```python
from build123d import *

# Parameters (mm, degrees)
F0_W     = 93.98
F0_H     = 38.1
F0_R     = 6.985
F1_DEPTH = 25.4
F3_D     = 5.5
F4_W     = 12.7
F4_H     = 5.08


with BuildPart() as f1:
    # F0 (on Front) → F1 (new body)
    with BuildSketch(Plane.XZ):
        with Locations((46.99, 19.05)):
            Rectangle(F0_W, F0_H)
        with Locations((15.24, 12.7)):
            Circle(F0_R, mode=Mode.SUBTRACT)
        Polygon((42.0011818976, 10.16), (50.8, 25.4), (59.5988181024, 10.16), align=None, mode=Mode.SUBTRACT)
    extrude(amount=F1_DEPTH)

    # F3 (through all)
    with Locations(Plane.XZ.offset(25.4)):
        with Locations((76.2, 25.4)):
            Hole(F3_D / 2)

    # F4 (on face) → F5 (revolve, cut)
    with BuildSketch(Plane.XY.offset(38.1)):
        with Locations((39.37, -15.24)):
            Rectangle(F4_W, F4_H)
    revolve(axis=Axis((46.99, 0, 38.1), (1, 0, 0)), mode=Mode.SUBTRACT)


solid = f1.part
```
Read the model definition and answer for the solid it produces. Units are mm, in the model's axes. A direction names the side the tool comes from. Coordinates: 2 decimals unless noted, no trailing zeros. Write each loop counter-clockwise with the first axis right and the second up, starting at its lowest first coordinate (ties: lowest second). Pieces come first, ordered by that corner, then holes. Notation, with made-up numbers: (60, 88) - (96, 88) arc R16 cw to (96, 97) - close; hole circle Ø5 at (88.5, 63). An arc over 180 degrees is marked (long way). Answer as a JSON object with one key per item and string values. Group by question number.
1. A cutting plane is placed at B-B (y = -22). Determine the outline of the cut face in (x, z) (3 decimals), plus the area to 3 significant figures.
2. This flat-tipped pin is pushed along its axis until it touches: P1, Ø11, axis at x = 15.24, z = 12.7, coming from the -Y side. Where does it stop, or does it pass through?
3. The mould has two halves that part along Y. Classify faces 4 (the flat face through (46.339, -12.522, 17.673)), 5 (the cylindrical face through (39.46, -9.08, 29.22)), 6 (the flat face through (46, -25.4, 19)), 7 (the cylindrical face through (39.459, -12.71, 25.667)): +Y half, -Y half, draft (parallel to the pull), parting line (faces both ways), or undercut.
4. A cutting plane is placed at A-A (x = 76.2). Determine the outline of the cut face in (y, z), plus the area to 3 significant figures.
5. Consider L1, parallel to Z at x = 15.24, y = -16.5 (3 decimals); L2, parallel to Z at x = 76.2, y = -8.25; L3, parallel to X at y = -9.25, z = 11. Determine where each line is inside the solid, lowest interval first. Write a range as [from, to].
6. A cutting plane is placed at C-C (z = 12.7). Determine the outline of the cut face in (x, y) (3 decimals), plus the area to 3 significant figures.
7. Which of the six approach directions +Z, -Z, +X, -X, +Y, -Y give full straight-line access (tool end or side, diameter ignored) to faces 1 (the flat face through (45.72, -11, 29)), 2 (the flat face through (51, -13, 10.16)), 3 (the flat face through (46, -13, 0))?
8. A cutting plane is placed at D-D (z = 7.5). Determine the outline of the cut face in (x, y).
Worked out:
{
 "1": {"outline": "(0, 0) - (93.98, 0) - (93.98, 38.1) - (0, 38.1) - close; hole circle Ø13.97 at (15.24, 12.7); hole (42.001, 10.16) - (59.599, 10.16) - (50.8, 25.4) - close; hole circle Ø5.5 at (76.2, 25.4)", "area": "3,270 mm²"},
 "2": {"P1": "passes through"},
 "3": {"face 4": "draft", "face 5": "undercut", "face 6": "-Y half", "face 7": "undercut"},
 "4": {"outline": "(-25.4, 0) - (0, 0) - (0, 22.65) - (-25.4, 22.65) - close; (-25.4, 28.15) - (0, 28.15) - (0, 38.1) - (-25.4, 38.1) - close", "area": "828 mm²"},
 "5": {"L1": "z = [0, 5.715], [19.685, 38.1]", "L2": "z = [0, 22.65], [28.15, 38.1]", "L3": "x = [0, 8.47], [22.01, 42.49], [59.11, 93.98]"},
 "6": {"outline": "(0, -25.4) - (8.255, -25.4) - (8.255, 0) - (0, 0) - close; (22.225, -25.4) - (43.468, -25.4) - (43.468, 0) - (22.225, 0) - close; (58.132, -25.4) - (93.98, -25.4) - (93.98, 0) - (58.132, 0) - close", "area": "1,660 mm²"},
 "7": {"face 1": "none", "face 2": "+Y, -Y", "face 3": "-Z, +X, -X, +Y, -Y"},
 "8": {"outline": "(0, -25.4) - (10.58, -25.4) - (10.58, 0) - (0, 0) - close; (19.9, -25.4) - (93.98, -25.4) - (93.98, 0) - (19.9, 0) - close"}
}
